from build123d import *

# Parameters (mm, degrees)
BOSS_EXTRUDE1_DEPTH = 116
SHELL1_T            = -3
FILLET1_R           = 1
CUT_EXTRUDE1_DEPTH  = 3


with BuildPart() as part:
    # Sketch1 → Boss-Extrude1 (new body)
    with BuildSketch(Plane(origin=(0, 0, 0), x_dir=(1, 0, 0), z_dir=(0, 1, 0))):
        with BuildLine():
            ThreePointArc((15.919007565, 0), (13, -15), (15.919007565, -30))
            Line((15.919007565, -30), (0, -30))
            Line((0, -30), (0, 0))
            Line((0, 0), (15.919007565, 0))
        make_face()
    extrude(amount=BOSS_EXTRUDE1_DEPTH)

    # Shell1
    shell1_openings = [part.faces().sort_by_distance(p)[0] for p in [
        (7.006000275, 116, 15),
        (7.006000275, 0, 15),
    ]]
    offset(amount=SHELL1_T, openings=shell1_openings, kind=Kind.INTERSECTION)

    # Fillet1
    fillet1_edges = [part.edges().sort_by_distance(p)[0] for p in [
        (0, 58, 30),
        (0, 58, 0),
    ]]
    fillet(fillet1_edges, radius=FILLET1_R)

    # Sketch2 → Cut-Extrude1 (cut)
    with BuildSketch(Plane.ZY):
        with BuildLine():
            Line((19, 96), (19, 20))
            ThreePointArc((19, 20), (15, 16), (11, 20))
            Line((11, 20), (11, 96))
            ThreePointArc((11, 96), (15, 100), (19, 96))
        make_face()
    extrude(amount=-CUT_EXTRUDE1_DEPTH, mode=Mode.SUBTRACT)


solid = part.part
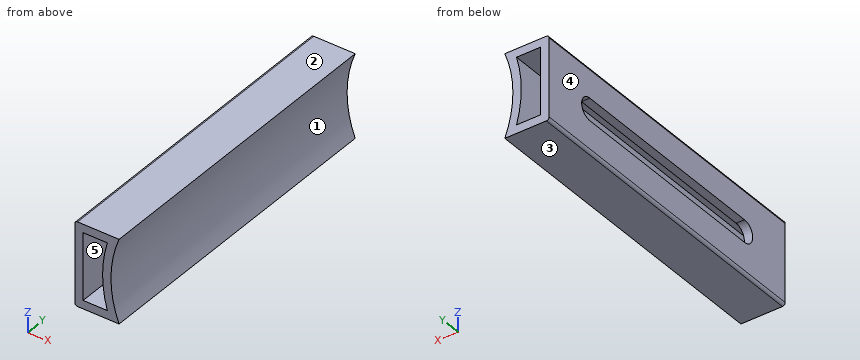
Could you check a few things on this model? Use its own coordinates, in mm. Face numbers are marked on the shaded views. A direction names the side the tool comes from. Round coordinates to 2 decimals unless told otherwise and drop trailing zeros. Loops run counter-clockwise (first coordinate to the right, second up) from the corner with the lowest first, then second, coordinate; pieces in that order, holes last. Notation, with made-up numbers: (-15, 88.5) - (6, 88.5) arc R20 ccw to (6, 105.5) - close; hole circle Ø5 at (56, 4). An arc over 180 degrees is marked (long way). Write item = value, one per line.
1) Imagine slicing it at D-D (y = 98.5). Please give me the cut outline in (x, z), and give its area (3 significant figures).
Computed:
outline = (0, 1) arc R1 ccw to (1, 0) - (15.92, 0) arc R40 cw to (15.92, 30) - (1, 30) arc R1 ccw to (0, 29) - (0, 18.12) - (3, 18.12) - (3, 27) - (11.71, 27) arc R43 ccw to (11.71, 3) - (3, 3) - (3, 11.88) - (0, 11.88) - close
area = 218 mm2
2) I need wall thicknesses on line 1 along Z through (x, y) = (2, 38); line 2 along X through (y, z) = (5.5, 14); line 3 along Z through (x, y) = (6.5, 18). Which ranges of each line are inside material? Lowest first, please. Write a range as from..to.
Computed:
line_1 = 0..11, 19..30
line_2 = 0..3, 10.01..13.01
line_3 = 0..3, 27..30
3) If we mould it in two halves opening along Z, with no side actions, what happens to the marked faces 1, 2 and 3? For each: pulls with the +Z half, pulls with the -Z half, needs draft (parallel to the pull), parting line crosses it, or undercut.
Computed:
face_1 = undercut
face_2 = pulls with the +Z half
face_3 = pulls with the -Z half
4) Imagine slicing it at A-A (x = 7.75). Please give me the cut outline in (y, z).
Computed:
outline = (0, 0) - (116, 0) - (116, 3) - (0, 3) - close; (0, 27) - (116, 27) - (116, 30) - (0, 30) - close
5) On a 3-axis mill with a long thin cutter (end or side, diameter ignored), from which of +Z, -Z, +X, -X, +Y, -Y can I reach the whole of each face in a straight line? I mean the marked faces 4 and 5. Say none if no direction works.
Computed:
face_4 = +Z, -Z, -X, +Y, -Y
face_5 = +Y, -Y
6) Imagine slicing it at C-C (y = 42.5). Please give me the cut outline in (x, z).
Computed:
outline = (0, 1) arc R1 ccw to (1, 0) - (15.92, 0) arc R40 cw to (15.92, 30) - (1, 30) arc R1 ccw to (0, 29) - (0, 19) - (3, 19) - (3, 27) - (11.71, 27) arc R43 ccw to (11.71, 3) - (3, 3) - (3, 11) - (0, 11) - close
7) Imagine slicing it at B-B (z = 15). Please give me the cut outline in (x, y), and give its area (3 significant figures).
Computed:
outline = (0, 0) - (3, 0) - (3, 16) - (0, 16) - close; (0, 100) - (3, 100) - (3, 116) - (0, 116) - close; (10, 0) - (13, 0) - (13, 116) - (10, 116) - close
area = 444 mm2
8) I'm going to push flat-ended pins straight in: P1, Ø6, axis at x = 9, z = 20, coming from the +Y side; P2, Ø5, axis at y = 37.5, z = 7.5, coming from the +X side. Where does each tip first touch, or does it pass through?
Computed:
P1 = 116
P2 = 14.27
